The listing builds one solid part. Answer for the finished solid, in the listing's coordinates (mm). Coordinates: 2 decimals unless noted, no trailing zeros. Write each loop counter-clockwise with the first axis right and the second up, starting at its lowest first coordinate (ties: lowest second). Pieces come first, ordered by that corner, then holes.
from build123d import *

# Parameters (mm, degrees)
F0_R     = 24
F0_R_2   = 23
F1_DEPTH = 9
F0_R_3   = 19
F2_DEPTH = 1
F3_R     = 0.49999


# Not quite as in the source:
# - a fillet or chamfer is up to 0.001 mm smaller than in the source, because OpenCascade refuses the exact size


with BuildPart() as f1:
    # F0 (on Top) → F1 (new body)
    with BuildSketch(Plane.XY):
        Circle(F0_R)
        Circle(F0_R_2, mode=Mode.SUBTRACT)
    extrude(amount=F1_DEPTH)

    # F0 (on Top) → F2 (join)
    with BuildSketch(Plane.XY):
        Circle(F0_R_2)
        Circle(F0_R_3, mode=Mode.SUBTRACT)
    extrude(amount=F2_DEPTH)

    # F3 (radius 0.5 in the source; OpenCascade refuses exactly that, so slightly less here)
    f3_edges = [f1.edges().sort_by_distance(p)[0] for p in [
        (-24, 0, 0),
        (-24, 0, 9),
        (-23, 0, 9),
    ]]
    fillet(f3_edges, radius=F3_R)


solid = f1.part
Q1. Determine the mould class of faces 1 (the face through (8.767, -16.856, 0.493)), 2 (the face through (-23.977, 1.055, 4.444)), 3 (the face through (-2.994, 22.804, 4.698)), 4 (the face through (9, -17, 0)) for opening direction X: released by +X, released by -X, zero draft, split by the parting line, or undercut.
Answers below:
face 1: undercut
face 2: split by the parting line
face 3: undercut
face 4: zero draft
Q2. The part is cut by section C-C, the plane z = 6. Write down the section's boundary in (x, y), then the cut area to 3 significant figures.
Answers below:
outline: circle Ø48 at (0, 0); hole circle Ø46 at (0, 0)
area: 148 mm2
Q3. Given pin 1 (1 mm diameter, centred on x = 4.5, z = 2.5, fed in from -Y); pin 2 (5 mm diameter, centred on y = 2.5, z = 5.5, fed in from -X); pin 3 (3 mm diameter, centred on x = -15, z = 4, fed in from +Y); pin 4 (12 mm diameter, centred on x = 2.5, y = 9.5, fed in from -Z), each flat-ended and moving along its own axis, determine where each tip first touches the part or whether it passes through.
Answers below:
pin 1: stops at y = -23.66
pin 2: stops at x = -24
pin 3: stops at y = 19.84
pin 4: passes through
Q4. Find the intervals of material crossed by probe 1 along Y at (x, z) = (0, 3.5); probe 2 along Y at (x, z) = (0, 0.55); probe 3 along Z at (x, y) = (9, -20), in increasing order.
Answers below:
probe 1: y = -24 to -23, 23 to 24
probe 2: y = -24 to -19, 19 to 24
probe 3: z = 0 to 1
